Can you work these out from the model? Positions are in its coordinate system, mm. A direction names the side the tool comes from. Round coordinates to 2 decimals unless told otherwise and drop trailing zeros. Order: outer loops, then holes, each group sorted by start corner. A loop starts at its lowest first (then second) coordinate and runs counter-clockwise, first axis right, second up.
Q1. If we section it at A-A (y = 4.75): Please give me the cut outline in (x, z).
Q2. We'd pull the mould along Z, two halves only. Please class faces 1 (the face through (10, 10, 60)), 2 (the face through (8, 10, 135)), 3 (the face through (5, 10, 150)), 4 (the face through (5, 10, 0)): pulls with the +Z half, pulls with the -Z half, needs draft (parallel to the pull), parting line crosses it, or undercut.
Q3. If we section it at B-B (z = 33): Please give me the cut outline in (x, y), plus the area to 3 significant figures.
Q4. Will these pins go through, and if not, where does the flat tip stop? P1, Ø5, axis at y = 10.5, z = 84.5, coming from the +X side; P2, Ø0.5, axis at x = 0.5, z = 113.5, coming from the -Y side.
Q5. If I drill on line 1 (Z direction, x = 9, y = 18.5); line 2 (X direction, y = 13.75, z = 18); line 3 (X direction, y = 8.25, z = 37), over which ranges is the centre line in solid material (lowest first)?
Q6. For faces 5 (the face through (8, 10, 35)), 6 (the face through (1, 10, 15)), 7 (the face through (10, 10, 15)), which set-ups out of +Z, -Z, +X, -X, +Y, -Y let a thin tool reach every point of the face, with its end or its side?
from build123d import *

# Parameters (mm, degrees)
F0_W     = 8
F0_H     = 20
F1_DEPTH = 150
F2_W     = 20
F2_H     = 9.75
F2_H_2   = 39.5
F2_H_3   = 29.75
F3_DEPTH = 2
F4_W     = 8
F4_H     = 10
F5_DEPTH = 1


with BuildPart() as f1:
    # F0 (on Top) → F1 (new body)
    with BuildSketch(Plane.XY):
        with Locations((4, 10)):
            Rectangle(F0_W, F0_H)
    extrude(amount=F1_DEPTH)

    # F2 (on face) → F3 (join)
    with BuildSketch(Plane.YZ.offset(8)):
        with Locations((10, 145.125)):
            Rectangle(F2_W, F2_H)
        with Locations((10, 110)):
            Rectangle(F2_W, F2_H_2)
        with Locations((10, 60)):
            Rectangle(F2_W, F2_H_2)
        with Locations((10, 14.875)):
            Rectangle(F2_W, F2_H_3)
    extrude(amount=F3_DEPTH)

    # F4 (on face) → F5 (cut)
    with BuildSketch(Plane(origin=(0, 0, 0), x_dir=(0, -1, 0), z_dir=(-1, 0, 0))):
        with Locations((-10, 115)):
            Rectangle(F4_W, F4_H)
        with Locations((-10, 65)):
            Rectangle(F4_W, F4_H)
        with Locations((-10, 15)):
            Rectangle(F4_W, F4_H)
    extrude(amount=-F5_DEPTH, mode=Mode.SUBTRACT)


solid = f1.part
Solution:
1. outline: (0, 0) - (10, 0) - (10, 29.75) - (8, 29.75) - (8, 40.25) - (10, 40.25) - (10, 79.75) - (8, 79.75) - (8, 90.25) - (10, 90.25) - (10, 129.75) - (8, 129.75) - (8, 140.25) - (10, 140.25) - (10, 150) - (0, 150) - close
2. face 1: needs draft
2. face 2: undercut
2. face 3: pulls with the +Z half
2. face 4: pulls with the -Z half
3. outline: (0, 0) - (8, 0) - (8, 20) - (0, 20) - close
3. area: 160 mm2
4. P1: stops at x = 8
4. P2: stops at y = 0
5. line 1: z = 0 to 29.75, 40.25 to 79.75, 90.25 to 129.75, 140.25 to 150
5. line 2: x = 1 to 10
5. line 3: x = 0 to 8
6. face 5: +X, +Y, -Y
6. face 6: -X
6. face 7: +Z, -Z, +X, +Y, -Y
